Can you work these out from the model? Positions are in its coordinate system, mm. Face numbers are marked on the shaded views. A direction names the side the tool comes from. Give positions to 0.01 mm unless a question says otherwise; leave off trailing zeros. Order: outer loops, then holes, each group sorted by start corner. A loop starts at its lowest first (then second) coordinate and runs counter-clockwise, first axis right, second up.
Item 1: I want a section at B-B, the plane y = 18. Write out the boundary of the cut face in (x, z).
Item 2: If I drill on line 1 along X through (y, z) = (3.85, -42.5); line 2 along Y through (x, z) = (5.5, -39); line 3 along X through (y, z) = (18, 24.25), over which ranges is the centre line in solid material (lowest first)?
Item 3: Which directions (+Z, -Z, +X, -X, +Y, -Y) give clear straight access to the entire face, cutting with the end or side of a thin tool? Please do the marked faces 1, 2, 3, 4 and 5.
Item 4: I want a section at A-A, the plane x = 0. Write out the boundary of the cut face in (y, z), then the cut area to 3 significant figures.
Item 5: I want a section at C-C, the plane z = 42.5. Write out the boundary of the cut face in (x, y), then the cut area to 3 significant figures.
Item 6: I want a section at D-D, the plane y = 4. Write out the boundary of the cut face in (x, z).
Item 7: I'm going to push flat-ended pins straight in: pin 1 Ø4.5 at (x, z) = (0, 42.5) entering from +Y; pin 2 Ø2.5 at (x, z) = (1.5, 24) entering from +Y; pin 3 Ø6 at (x, y) = (-6, 14.5) entering from +Z. Where does each tip first touch, or does it pass through?
Item 8: If we mould it in two halves opening along Y, with no side actions, what happens to the marked faces 6, 7 and 8? For each: +Y half, -Y half, draft (parallel to the pull), parting line (faces both ways), or undercut.
```python
from build123d import *

# Parameters (mm, degrees)
ESBO_O1_W                = 8
ESBO_O1_H                = 2
RESSALTO_EXTRUS_O1_DEPTH = 10
CORTE_EXTRUS_O1_REACH    = 75.763
ESBO_O4_W                = 20
ESBO_O4_H                = 15
ESBO_O4_R                = 2
RESSALTO_EXTRUS_O2_DEPTH = 5


with BuildPart() as part:
    # Esboço1 → Ressalto-extrusão1 (new, symmetric)
    with BuildSketch(Plane(origin=(0, 0, 0), x_dir=(0, 0, -1), z_dir=(1, 0, 0))):
        Polygon((-35, 21), (-10, 21), (-10, 5), (10, 5), (10, 21), (35, 21), (35, 0), (-35, 0), align=None)
        with Locations((-22.5, 4)):
            Rectangle(ESBO_O1_W, ESBO_O1_H, mode=Mode.SUBTRACT)
        with Locations((22.5, 4)):
            Rectangle(ESBO_O1_W, ESBO_O1_H, mode=Mode.SUBTRACT)
    extrude(amount=RESSALTO_EXTRUS_O1_DEPTH, both=True)

    # Corte-extrusão1: up to this face of the body (flat: up to its plane)
    corte_extrus_o1_end = Plane(part.part.faces().sort_by_distance((0, 10.5, -35))[0])
    # Esboço2 → Corte-extrusão1 (cut, up to the picked face)
    with BuildSketch(Plane.XY.offset(35), mode=Mode.PRIVATE) as corte_extrus_o1_sk1:
        with BuildLine():
            Line((-6.873863542, 21), (6.873863542, 21))
            ThreePointArc((6.873863542, 21), (0, 10.5), (-6.873863542, 21))
        make_face()
    corte_extrus_o1_tool1 = split(extrude(corte_extrus_o1_sk1.sketch, amount=-CORTE_EXTRUS_O1_REACH, mode=Mode.PRIVATE), bisect_by=corte_extrus_o1_end, keep=Keep.BOTH, mode=Mode.PRIVATE)
    add(corte_extrus_o1_tool1.solids().sort_by(Axis((0, 16.361219, 35), (0, 0, -1)))[0], mode=Mode.SUBTRACT)

    # Esboço4 → Ressalto-extrusão2 (add)
    # profile 1 of 2: a face of its own
    with BuildSketch(Plane(origin=(0, 5, 0), x_dir=(1, 0, 0), z_dir=(0, 1, 0))):
        with Locations((0, 42.5)):
            Rectangle(ESBO_O4_W, ESBO_O4_H)
        with Locations(Location((0, 42.5, 0), (0, 0, 270))):
            Circle(ESBO_O4_R, mode=Mode.SUBTRACT)
    # profile 2 of 2: a face of its own
    with BuildSketch(Plane(origin=(0, 5, 0), x_dir=(1, 0, 0), z_dir=(0, 1, 0))):
        with Locations((0, -42.5)):
            Rectangle(ESBO_O4_W, ESBO_O4_H)
        with Locations(Location((0, -42.5, 0), (0, 0, 270))):
            Circle(ESBO_O4_R, mode=Mode.SUBTRACT)
    extrude(amount=-RESSALTO_EXTRUS_O2_DEPTH)


solid = part.part
```
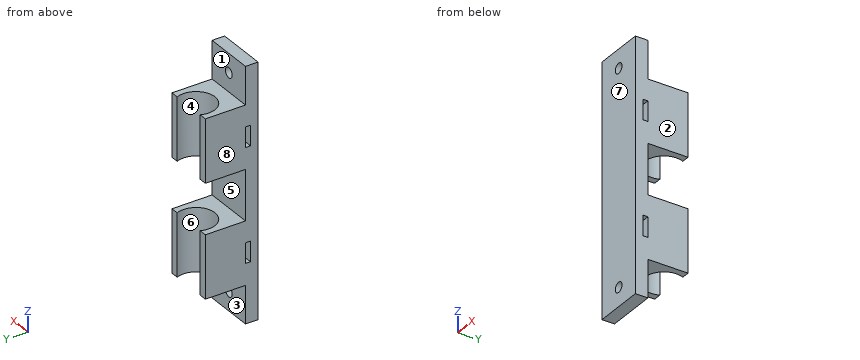
Results list:
1. outline: (-10, -35) - (-7.5, -35) - (-7.5, -10) - (-10, -10) - close; (-10, 10) - (-7.5, 10) - (-7.5, 35) - (-10, 35) - close; (7.5, -35) - (10, -35) - (10, -10) - (7.5, -10) - close; (7.5, 10) - (10, 10) - (10, 35) - (7.5, 35) - close
2. line 1: x = -10 to -2, 2 to 10
2. line 2: y = 0 to 5
2. line 3: x = -10 to -7.5, 7.5 to 10
3. face 1: +Z, +X, -X, +Y
3. face 2: +Z, -Z, +X, +Y, -Y
3. face 3: -Z, +X, -X, +Y
3. face 4: +Z, -Z
3. face 5: +X, -X, +Y
4. outline: (0, -50) - (5, -50) - (5, -44.5) - (0, -44.5) - close; (0, -40.5) - (5, -40.5) - (5, -35) - (10.5, -35) - (10.5, -10) - (5, -10) - (5, 10) - (10.5, 10) - (10.5, 35) - (5, 35) - (5, 40.5) - (0, 40.5) - close; (0, 44.5) - (5, 44.5) - (5, 50) - (0, 50) - close; hole (3, -26.5) - (5, -26.5) - (5, -18.5) - (3, -18.5) - close; hole (3, 18.5) - (5, 18.5) - (5, 26.5) - (3, 26.5) - close
4. area: 703 mm2
5. outline: (-10, 0) - (-2, 0) - (-2, 5) - (-10, 5) - close; (2, 0) - (10, 0) - (10, 5) - (2, 5) - close
5. area: 80.0 mm2
6. outline: (-10, -50) - (10, -50) - (10, -26.5) - (-10, -26.5) - close; (-10, -18.5) - (10, -18.5) - (10, 18.5) - (-10, 18.5) - close; (-10, 26.5) - (10, 26.5) - (10, 50) - (-10, 50) - close; hole circle Ø4 at (0, -42.5); hole circle Ø4 at (0, 42.5)
7. pin 1: stops at y = 5
7. pin 2: stops at y = 11.02
7. pin 3: stops at z = 35
8. face 6: undercut
8. face 7: -Y half
8. face 8: draft
